Autodesk Inventor part; units mm, degrees
ref_plane "YZ Plane" through (0, 0, 0) normal (1, 0, 0) x (0, 1, 0)
ref_plane "XZ Plane" through (0, 0, 0) normal (0, 1, 0) x (-1, 0, 0)
ref_plane "XY Plane" through (0, 0, 0) normal (0, 0, 1) x (1, 0, 0)
sketch "Sketch1" plane through (0, 0, 0) normal (0, 0, 1) x (1, 0, 0)
  line L0 (0, 0) -> (28.575, 0)
  line L1 (82.55, 0) -> (82.55, 57.15)
  line L2 (82.55, 57.15) -> (53.975, 57.15)
  line L3 (0, 57.15) -> (0, 0)
  line L4 (0, 53.975) -> (28.575, 53.975) construction
  line L5 (28.575, 57.15) -> (28.575, 53.975)
  line L6 (53.975, 57.15) -> (53.975, 53.975)
  line L7 (53.975, 53.975) -> (82.55, 53.975) construction
  line L8 (28.575, 53.975) -> (53.975, 53.975)
  line L9 (53.975, 57.15) -> (28.575, 57.15) construction
  line L10 (28.575, 57.15) -> (0, 57.15)
  line L11 (0, 3.175) -> (28.575, 3.175) construction
  line L12 (53.975, 0) -> (53.975, 3.175)
  line L13 (28.575, 0) -> (28.575, 3.175)
  line L14 (28.575, 0) -> (53.975, 0) construction
  line L15 (53.975, 0) -> (82.55, 0)
  line L16 (53.975, 3.175) -> (82.55, 3.175) construction
  line L17 (28.575, 3.175) -> (53.975, 3.175)
  dimension "d0" = 82.55
  dimension "d1" = 57.15
  dimension "d2" = 28.575
  dimension "d3" = 25.4
  dimension "d4" = 3.175
  dimension "d5" = 3.175
  dimension "d6" = 28.575
  dimension "d7" = 25.4
extrude "Extrusion1" add sketch "Sketch1" along normal blind 3.175
sketch "Sketch4" plane through (0, 0, 3.175) normal (0, 0, 1) x (1, 0, 0)
  line L0 (82.55, 0) -> (82.55, 57.15)
  line L1 (53.975, 53.975) -> (28.575, 53.975)
  line L2 (0, 57.15) -> (0, 0)
  line L3 (28.575, 3.175) -> (53.975, 3.175)
  line L4 (28.575, 3.175) -> (0, 3.175)
  line L5 (0, 3.175) -> (0, 0)
  line L6 (0, 0) -> (28.575, 0)
  line L7 (28.575, 0) -> (28.575, 3.175)
  line L8 (53.975, 3.175) -> (82.55, 3.175)
  line L9 (82.55, 3.175) -> (82.55, 0)
  line L10 (82.55, 0) -> (53.975, 0)
  line L11 (53.975, 0) -> (53.975, 3.175)
  line L12 (53.975, 53.975) -> (82.55, 53.975)
  line L13 (82.55, 53.975) -> (82.55, 57.15)
  line L14 (82.55, 57.15) -> (53.975, 57.15)
  line L15 (53.975, 57.15) -> (53.975, 53.975)
  line L16 (28.575, 53.975) -> (0, 53.975)
  line L17 (0, 53.975) -> (0, 57.15)
  line L18 (0, 57.15) -> (28.575, 57.15)
  line L19 (28.575, 57.15) -> (28.575, 53.975)
  line L20 (0, 28.575) -> (82.55, 28.575) construction
  line L21 (41.275, 53.975) -> (41.275, 3.175) construction
  line L22 (23.775, 47.2281) -> (58.775, 47.2281) construction
  line L23 (58.775, 47.2281) -> (58.775, 9.9219) construction
  line L24 (58.775, 9.9219) -> (23.775, 9.9219) construction
  line L25 (23.775, 9.9219) -> (23.775, 47.2281) construction
  line L26 (0, 27.3573) -> (82.55, 27.3573) construction
  line L27 (82.55, 12.3573) -> (0, 12.3573) construction
  line L28 (6.35, 8.7312) -> (76.2, 8.7312)
  line L29 (76.2, 8.7312) -> (76.2, 11.9062)
  line L30 (76.2, 11.9062) -> (6.35, 11.9062)
  line L31 (6.35, 11.9062) -> (6.35, 8.7312)
  line L32 (0, 19.8573) -> (82.55, 19.8573) construction
  line L33 (76.2, 27.8083) -> (76.2, 30.9833)
  line L34 (76.2, 30.9833) -> (6.35, 30.9833)
  line L35 (6.35, 30.9833) -> (6.35, 27.8083)
  line L36 (6.35, 27.8083) -> (76.2, 27.8083)
  dimension "d39" = 35
  dimension "d40" = 37.3062
  dimension "d41" = 15
  dimension "d42" = 2.4354
  dimension "d43" = 69.85
  dimension "d44" = 3.175
  dimension "d45" = 5.5563
  dimension "d46" = 0.451
  dimension "d47" = 69.85
extrude "Extrusion4" add sketch "Sketch4" along normal blind 12.7 contours L10 L11 L8 L0 | L12 L15 L14 L0 | L7 L6 L2 L4 | L16 L2 L18 L19 | L31 L30 L29 L28 | L36 L35 L34 L33
equation "\"d2\" = -0.5 * d3 + 0.5 * d0"
equation "\"d6\" = d2"
equation "\"d7\" = d3"
equation "\"d42\" = -0.666667 * d41 + 0.333333 * d40"
equation "\"d43\" = d47"
properties part number "Belt Aligners" material "Polyethylene, High Density"
Read the model definition and answer for the solid it produces. Units are mm, in the model's axes. A direction names the side the tool comes from. Round coordinates to 2 decimals unless told otherwise and drop trailing zeros. Loops run counter-clockwise (first coordinate to the right, second up) from the corner with the lowest first, then second, coordinate; pieces in that order, holes last. Notation, with made-up numbers: (34, 6) -> (79, 6) arc R13 ccw to (79, 30) -> close; hole circle Ø4 at (-12, -20). An arc over 180 degrees is marked (long way). One line per item, written item: value.
1) A cutting plane is placed at C-C (y = 50). Determine the outline of the cut face in (x, z) (3 decimals), and give its area (3 significant figures).
Answer list:
outline: (0, 0) -> (82.55, 0) -> (82.55, 3.175) -> (0, 3.175) -> close
area: 262 mm²
2) Consider L1, parallel to Y at x = 10, z = 15.25 (3 decimals); L2, parallel to Y at x = 47, z = 5.25; L3, parallel to X at y = 54.5, z = 6 (3 decimals). Determine where each line is inside the solid, lowest interval first. Write a range as [from, to].
Answer list:
L1: y = [0, 3.175], [8.731, 11.906], [27.808, 30.983], [53.975, 57.15]
L2: y = [8.73, 11.91], [27.81, 30.98]
L3: x = [0, 28.575], [53.975, 82.55]
3) A cutting plane is placed at B-B (x = 53). Determine the outline of the cut face in (y, z) (3 decimals), and give its area (3 significant figures).
Answer list:
outline: (3.175, 0) -> (53.975, 0) -> (53.975, 3.175) -> (30.983, 3.175) -> (30.983, 15.875) -> (27.808, 15.875) -> (27.808, 3.175) -> (11.906, 3.175) -> (11.906, 15.875) -> (8.731, 15.875) -> (8.731, 3.175) -> (3.175, 3.175) -> close
area: 242 mm²
4) For faces 4 (the face through (28.575, 2, 8)), 5 (the face through (14, 53.975, 9)), 6 (the face through (6.35, 10, 9)), determine the directions among +Z, -Z, +X, -X, +Y, -Y from which every point of the face is accessible in a straight line to the end or side of a thin tool.
Answer list:
face 4: +Z, -Z, -Y
face 5: +Z, +X, -X
face 6: +Z, -X
5) A cutting plane is placed at A-A (z = 13.5). Determine the outline of the cut face in (x, y) (3 decimals), and give its area (3 significant figures).
Answer list:
outline: (0, 0) -> (28.575, 0) -> (28.575, 3.175) -> (0, 3.175) -> close; (0, 53.975) -> (28.575, 53.975) -> (28.575, 57.15) -> (0, 57.15) -> close; (6.35, 8.731) -> (76.2, 8.731) -> (76.2, 11.906) -> (6.35, 11.906) -> close; (6.35, 27.808) -> (76.2, 27.808) -> (76.2, 30.983) -> (6.35, 30.983) -> close; (53.975, 0) -> (82.55, 0) -> (82.55, 3.175) -> (53.975, 3.175) -> close; (53.975, 53.975) -> (82.55, 53.975) -> (82.55, 57.15) -> (53.975, 57.15) -> close
area: 806 mm²
6) Flat-ended cylindrical pins translate along their axes: P1, Ø1, axis at x = 28, y = 39.5, coming from the +Z side (3 decimals); P2, Ø1.6, axis at y = 30, z = 12.5, coming from the -X side; P3, Ø1, axis at x = 36.5, z = 1, coming from the -Y side (3 decimals); P4, Ø1, axis at y = 24.5, z = 5.5, coming from the -X side. Find the tip coordinate at first contact, or state that the pin passes through.
Answer list:
P1: stops at z = 3.175
P2: stops at x = 6.35
P3: stops at y = 3.175
P4: passes through
7) A cutting plane is placed at D-D (x = 9). Determine the outline of the cut face in (y, z) (3 decimals), and give its area (3 significant figures).
Answer list:
outline: (0, 0) -> (57.15, 0) -> (57.15, 15.875) -> (53.975, 15.875) -> (53.975, 3.175) -> (30.983, 3.175) -> (30.983, 15.875) -> (27.808, 15.875) -> (27.808, 3.175) -> (11.906, 3.175) -> (11.906, 15.875) -> (8.731, 15.875) -> (8.731, 3.175) -> (3.175, 3.175) -> (3.175, 15.875) -> (0, 15.875) -> close
area: 343 mm²
8) The mould has two halves that part along Y. Classify faces 1 (the face through (41, 23, 3.175)), 2 (the face through (82.55, 26, 2)), 3 (the face through (41, 53.975, 2)): pulls with the +Y half, pulls with the -Y half, needs draft (parallel to the pull), parting line crosses it, or undercut.
Answer list:
face 1: undercut
face 2: needs draft
face 3: pulls with the +Y half
